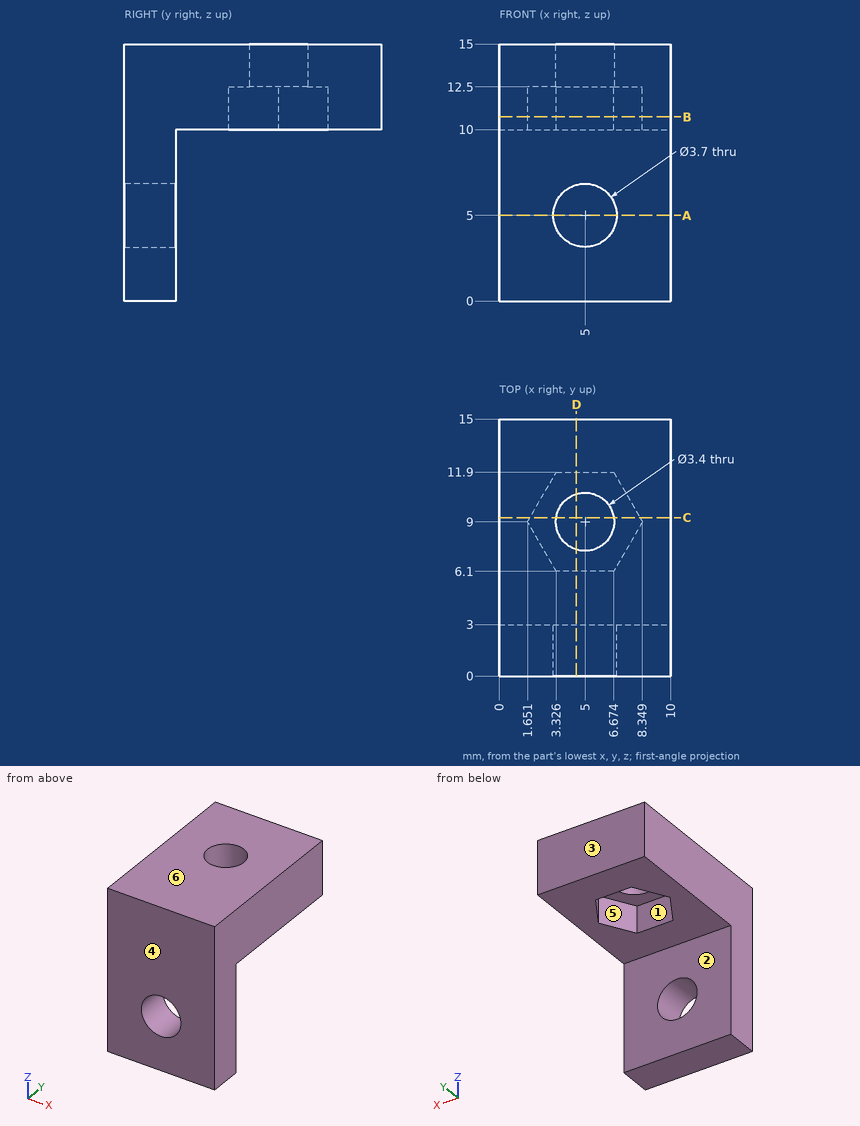
Here's the drawing with two shaded views (mm, measured from the low corner). I have some questions. A direction names the side the tool comes from. Give positions to 0.01 mm unless a question says otherwise; leave off trailing zeros. Order: outer loops, then holes, each group sorted by start corner. A loop starts at its lowest first (then second) coordinate and runs counter-clockwise, first axis right, second up.
Q1. Suppose I cut it at C-C, the plane y = 9.25. Write out the boundary of the cut face in (x, z) (1 decimal).
Q2. Suppose I cut it at A-A, the plane z = 5. Write out the boundary of the cut face in (x, y).
Q3. I'm going to push flat-ended pins straight in: P1, Ø3, axis at x = 5.5, y = 7.5, coming from the -Z side; P2, Ø2, axis at x = 3, z = 5.5, coming from the +Y side; P3, Ø3, axis at x = 4.5, y = 8.5, coming from the -Z side. Where does each tip first touch, or does it pass through?
Q4. We'd pull the mould along Y, two halves only. Please class the marked faces 4, 5 and 6: +Y half, -Y half, draft (parallel to the pull), parting line (faces both ways), or undercut.
Q5. For the marked faces 1, 2 and 3, which set-ups out of +Z, -Z, +X, -X, +Y, -Y let a thin tool reach every point of the face, with its end or its side?
Q6. If I drill on line 1 along Y through (x, z) = (5, 14.05); line 2 along Y through (x, z) = (4.75, 2.75); line 3 along X through (y, z) = (1.75, 5), over which ranges is the centre line in solid material (lowest first)?
Q7. Suppose I cut it at D-D, the plane x = 4.5. Write out the boundary of the cut face in (y, z) (1 decimal).
Q8. Suppose I cut it at B-B, the plane z = 10.75. Write out the boundary of the cut face in (x, y) (1 decimal), and give its area (3 significant figures).
Solution:
1. outline: (0, 10) - (1.8, 10) - (1.8, 12.5) - (3.3, 12.5) - (3.3, 15) - (0, 15) - close; (6.7, 12.5) - (8.2, 12.5) - (8.2, 10) - (10, 10) - (10, 15) - (6.7, 15) - close
2. outline: (0, 0) - (3.15, 0) - (3.15, 3) - (0, 3) - close; (6.85, 0) - (10, 0) - (10, 3) - (6.85, 3) - close
3. P1: stops at z = 10
3. P2: stops at y = 3
3. P3: stops at z = 12.5
4. face 4: -Y half
4. face 5: undercut
4. face 6: draft
5. face 1: -Z
5. face 2: -Z, +X, -X, +Y
5. face 3: +Z, -Z, +X, -X, +Y
6. line 1: y = 0 to 7.3, 10.7 to 15
6. line 2: y = 0 to 3
6. line 3: x = 0 to 3.15, 6.85 to 10
7. outline: (0, 0) - (3, 0) - (3, 3.2) - (0, 3.2) - close; (0, 6.8) - (3, 6.8) - (3, 10) - (6.1, 10) - (6.1, 12.5) - (7.4, 12.5) - (7.4, 15) - (0, 15) - close; (10.6, 12.5) - (11.9, 12.5) - (11.9, 10) - (15, 10) - (15, 15) - (10.6, 15) - close
8. outline: (0, 0) - (10, 0) - (10, 15) - (0, 15) - close; hole (1.7, 9) - (3.3, 6.1) - (6.7, 6.1) - (8.3, 9) - (6.7, 11.9) - (3.3, 11.9) - close
8. area: 121 mm2
